Work out the finished part from the listing and answer in its coordinate system (mm). A direction names the side the tool comes from. Round coordinates to 2 decimals unless told otherwise and drop trailing zeros. Write each loop counter-clockwise with the first axis right and the second up, starting at its lowest first coordinate (ties: lowest second). Pieces come first, ordered by that corner, then holes.
1. Find section A-A (z = 4.25). Write down the section's boundary in (x, y), and give its area (3 significant figures).
2. Find section C-C (x = 255.5). Write down the section's boundary in (y, z), and give its area (3 significant figures).
3. Flat-ended cylindrical pins translate along their axes: pin 1 Ø1.5 at (y, z) = (115, 1) entering from +X; pin 2 Ø6.5 at (x, y) = (-132, -47) entering from +Z; pin 3 Ø1.5 at (y, z) = (-214.5, 7) entering from +X. Find the tip coordinate at first contact, or state that the pin passes through.
4. Find section D-D (y = 0). Write down the section's boundary in (x, z), and give its area (3 significant figures).
5. Determine the mould class of faces 1 (the face through (359.913, -7.916, 3.944)), 2 (the face through (349.915, -7.696, 0.986)), 3 (the face through (70, 5, 0)) for opening direction X: pulls with the +X half, pulls with the -X half, needs draft (parallel to the pull), parting line crosses it, or undercut.
6. A tool of negligible diameter and unlimited length cuts with its end or side. For faces 4 (the face through (351.915, 7.74, 0.986)), 5 (the face through (-163, -48, 2)), 6 (the face through (348, 55, 0)), from which of +Z, -Z, +X, -X, +Y, -Y can it reach the whole face along a straight path? Write none if from no direction.
7. Straight lines are drawn through the part: probe 1 along Y at (x, z) = (-132, 3.5); probe 2 along Y at (x, z) = (169.5, 1.25); probe 3 along X at (y, z) = (-83.5, 2.75). For each, find the intervals that lie inside material, in ascending order.
8. Find section B-B (y = 128). Write down the section's boundary in (x, z).
```python
from build123d import *

# Parameters (mm, degrees)
F1_DEPTH = 8
F3_DEPTH = 2
F4_R     = 4
F5_DEPTH = 8
F7_DEPTH = 2


with BuildPart() as f1:
    # F0 (on Top) → F1 (new body)
    with BuildSketch(Plane.XY):
        with BuildLine():
            Line((-202, -360), (0, -360))
            ThreePointArc((0, -360), (360, 0), (0, 360))
            Line((0, 360), (-202, 360))
            Line((-202, 360), (-202, -360))
        make_face()
    extrude(amount=F1_DEPTH)

    # F2 (on face) → F3 (cut)
    with BuildSketch(Plane(origin=(0, 0, 0), x_dir=(1, 0, 0), z_dir=(0, 0, -1))):
        with BuildLine():
            ThreePointArc((0, 350), (350, 0), (0, -350))
            Line((0, -350), (-202, -350))
            Line((-202, -350), (-202, -352))
            Line((-202, -352), (0, -352))
            ThreePointArc((0, -352), (352, 0), (0, 352))
            Line((0, 352), (-202, 352))
            Line((-202, 352), (-202, 350))
            Line((-202, 350), (0, 350))
        make_face()
    extrude(amount=-F3_DEPTH, mode=Mode.SUBTRACT)

    # F4 (on face) → F5 (cut, through all)
    with BuildSketch(Plane.XY.offset(8)):
        with Locations((-132, -47)):
            Circle(F4_R)
    extrude(amount=-F5_DEPTH, mode=Mode.SUBTRACT)

    # F6 (on face) → F7 (cut)
    with BuildSketch(Plane(origin=(0, 0, 0), x_dir=(1, 0, 0), z_dir=(0, 0, -1))):
        with BuildLine():
            Line((-202, 149), (-202, -55))
            ThreePointArc((-202, -55), (-100, 47), (-202, 149))
        make_face()
    extrude(amount=-F7_DEPTH, mode=Mode.SUBTRACT)


solid = f1.part
```
Worked answers:
1. outline: (-202, -360) - (0, -360) arc R360 ccw to (0, 360) - (-202, 360) - close; hole circle Ø8 at (-132, -47)
1. area: 349,000 mm2
2. outline: (-253.61, 0) - (-242.12, 0) - (-242.12, 2) - (-239.21, 2) - (-239.21, 0) - (239.21, 0) - (239.21, 2) - (242.12, 2) - (242.12, 0) - (253.61, 0) - (253.61, 8) - (-253.61, 8) - close
2. area: 4,050 mm2
3. pin 1: stops at x = 341.39
3. pin 2: passes through
3. pin 3: stops at x = 289.67
4. outline: (-202, 2) - (-111.47, 2) - (-111.47, 0) - (350, 0) - (350, 2) - (352, 2) - (352, 0) - (360, 0) - (360, 8) - (-202, 8) - close
4. area: 4,310 mm2
5. face 1: pulls with the +X half
5. face 2: undercut
5. face 3: needs draft
6. face 4: -Z
6. face 5: -Z, -X
6. face 6: -Z, +X, -X, +Y, -Y
7. probe 1: y = -360 to -51, -43 to 360
7. probe 2: y = -317.6 to -308.5, -306.22 to 306.22, 308.5 to 317.6
7. probe 3: x = -202 to 350.18
8. outline: (-202, 0) - (325.75, 0) - (325.75, 2) - (327.9, 2) - (327.9, 0) - (336.48, 0) - (336.48, 8) - (-202, 8) - close
